Design review of the part built by this model. Coordinates are the model's own, in mm. A direction names the side the tool comes from. Coordinates: 2 decimals unless noted, no trailing zeros. Loops run counter-clockwise (first coordinate to the right, second up) from the corner with the lowest first, then second, coordinate; pieces in that order, holes last. Notation, with made-up numbers: (62, 10) -> (70, 10) arc R20 cw to (70, 49) -> close; hole circle Ø6 at (-11.75, 65.25). An arc over 180 degrees is marked (long way). Use CSV: the item, a comma, the result in double quotes.
```python
from build123d import *

# Parameters (mm, degrees)
BOSS_EXTRUDE1_DEPTH = 15
FILLET1_R           = 5
SKETCH2_W           = 8
SKETCH2_H           = 15
CUT_EXTRUDE1_DEPTH  = 100
SKETCH3_W           = 15
SKETCH3_H           = 70
CUT_EXTRUDE3_DEPTH  = 100
CUT_EXTRUDE4_DEPTH  = 3.75
SKETCH9_R           = 2.5
CUT_EXTRUDE5_DEPTH  = 7.5
SKETCH10_W          = 2.5
SKETCH10_H          = 90
CUT_EXTRUDE6_DEPTH  = 218.431134071
FILLET2_R           = 2
BOSS_EXTRUDE2_DEPTH = 19
SKETCH12_W          = 13.011456799
SKETCH12_H          = 10.932703346
CUT_EXTRUDE7_DEPTH  = 7


with BuildPart() as part:
    # Sketch1 → Boss-Extrude1 (new body)
    with BuildSketch(Plane.XY):
        with BuildLine():
            Line((-15, -103.255813953), (-15, 136.744186047))
            ThreePointArc((-15, 136.744186047), (0, 151.744186047), (15, 136.744186047))
            Line((15, 136.744186047), (140, 136.744186047))
            Line((140, 136.744186047), (140, 111.744186047))
            Line((140, 111.744186047), (15, 111.744186047))
            Line((15, 111.744186047), (15, -103.255813953))
            ThreePointArc((15, -103.255813953), (0, -118.255813953), (-15, -103.255813953))
        make_face()
    extrude(amount=BOSS_EXTRUDE1_DEPTH)

    # Fillet1
    fillet1_edges = [part.edges().sort_by_distance(p)[0] for p in [
        (0, -118.255813953, 0),
        (77.5, 111.744186047, 15),
        (77.5, 136.744186047, 15),
        (0, 151.744186047, 15),
        (-15, 16.744186047, 15),
        (0, -118.255813953, 15),
        (-15, 16.744186047, 0),
        (0, 151.744186047, 0),
        (77.5, 136.744186047, 0),
        (15, 4.244186047, 15),
        (77.5, 111.744186047, 0),
        (15, 4.244186047, 0),
    ]]
    fillet(fillet1_edges, radius=FILLET1_R)

    # Sketch2 → Cut-Extrude1 (cut)
    with BuildSketch(Plane(origin=(140, 0, 0), x_dir=(0, 0, -1), z_dir=(1, 0, 0))):
        with Locations((-7.5, 124.244186047)):
            Rectangle(SKETCH2_W, SKETCH2_H)
    extrude(amount=-CUT_EXTRUDE1_DEPTH, mode=Mode.SUBTRACT)

    # Sketch3 → Cut-Extrude3 (cut)
    with BuildSketch(Plane.XY.offset(15)):
        with Locations((0, -83.255813953)):
            Rectangle(SKETCH3_W, SKETCH3_H)
    extrude(amount=-CUT_EXTRUDE3_DEPTH, mode=Mode.SUBTRACT)

    # Sketch6 → Revolve1 (revolve)
    with BuildSketch(Plane.XY.offset(7.5)):
        with BuildLine():
            Line((-7.5, -101.255813953), (-5.5, -101.255813953))
            ThreePointArc((-5.5, -101.255813953), (-6.085786438, -99.841600391), (-7.5, -99.255813953))
            Line((-7.5, -99.255813953), (-7.5, -101.255813953))
        make_face()
        with BuildLine():
            Line((7.5, -101.255813953), (5.5, -101.255813953))
            ThreePointArc((5.5, -101.255813953), (6.085786438, -99.841600391), (7.5, -99.255813953))
            Line((7.5, -99.255813953), (7.5, -101.255813953))
        make_face()
    revolve(axis=Axis((22.79505848, -101.255813953, 7.5), (-1, 0, 0)))

    # Sketch8 → Cut-Extrude4 (cut, symmetric)
    with BuildSketch(Plane(origin=(0, 0, 0), x_dir=(0, 0, -1), z_dir=(1, 0, 0))):
        Polygon((-7.5, 91.744186047), (0, 86.49262951), (0, 76.49262951), (-7.5, 81.744186047), align=None)
        Polygon((0, 56.49262951), (0, 66.49262951), (-7.5, 71.744186047), (-7.5, 61.744186047), align=None)
        Polygon((0, 36.49262951), (0, 46.49262951), (-7.5, 51.744186047), (-7.5, 41.744186047), align=None)
    extrude(amount=CUT_EXTRUDE4_DEPTH, both=True, mode=Mode.SUBTRACT)

    # Sketch9 → Cut-Extrude5 (cut)
    with BuildSketch(Plane(origin=(0, 0, 0), x_dir=(-1, 0, 0), z_dir=(0, 0, -1))):
        with Locations((-130, 124.244186047)):
            Circle(SKETCH9_R)
        with Locations((-110, 124.244186047)):
            Circle(SKETCH9_R)
        with Locations((-90, 124.244186047)):
            Circle(SKETCH9_R)
        with Locations((-70, 124.244186047)):
            Circle(SKETCH9_R)
        with Locations((-50, 124.244186047)):
            Circle(SKETCH9_R)
    extrude(amount=-CUT_EXTRUDE5_DEPTH, mode=Mode.SUBTRACT)

    # Sketch10 → Cut-Extrude6 (cut, through all)
    with BuildSketch(Plane.ZY.offset(15)):
        with Locations((1.25, -38.255813953)):
            Rectangle(SKETCH10_W, SKETCH10_H)
    extrude(amount=-CUT_EXTRUDE6_DEPTH, mode=Mode.SUBTRACT)

    # Fillet2
    fillet2_edges = [part.edges().sort_by_distance(p)[0] for p in [
        (-12.5, 6.744186047, 0.669872981),
        (12.5, 6.744186047, 0.669872981),
        (8.75, -83.255813953, 0),
        (-8.75, -83.255813953, 0),
        (12.5, -83.255813953, 0.669872981),
        (-12.5, -83.255813953, 0.669872981),
        (0, 6.744186047, 0),
    ]]
    fillet(fillet2_edges, radius=FILLET2_R)

    # Sketch11 → Boss-Extrude2 (add)
    with BuildSketch(Plane.ZY.offset(15)):
        with BuildLine():
            Line((0, 109.244186047), (0, 101.244186047))
            ThreePointArc((0, 101.244186047), (-0.878679656, 103.36550639), (-3, 104.244186047))
            Line((-3, 104.244186047), (-7, 104.244186047))
            Line((-7, 104.244186047), (-7, 109.244186047))
            Line((-7, 109.244186047), (0, 109.244186047))
        make_face()
    extrude(amount=-BOSS_EXTRUDE2_DEPTH)

    # Sketch12 → Cut-Extrude7 (cut)
    with BuildSketch(Plane(origin=(0, 0, -7), x_dir=(-1, 0, 0), z_dir=(0, 0, -1))):
        with Locations((10.2557284, 106.179286635)):
            Rectangle(SKETCH12_W, SKETCH12_H)
    extrude(amount=-CUT_EXTRUDE7_DEPTH, mode=Mode.SUBTRACT)


solid = part.part
```
Item 1: Clearance check with flat-ended pins moving along their axes: pin 1 (4 mm diameter, centred on y = -66, z = 4, fed in from +X); pin 2 (2.5 mm diameter, centred on x = 91.5, z = 6.5, fed in from -Y); pin 3 (3.5 mm diameter, centred on y = 103.5, z = -4, fed in from +X). State where each tip first meets the part, or that it passes through.
Checked values:
pin 1,"x = 15"
pin 2,"y = 111.74"
pin 3,"x = 4"
Item 2: Draft analysis for pull direction Z (two halves, no side actions). For faces 5 (the face through (70.325, 126.723, 1.726)), 6 (the face through (3.75, 44, 4)), 7 (the face through (74.09, 113.17, 1.504)), state which applies: pulls with the +Z half, pulls with the -Z half, needs draft (parallel to the pull), parting line crosses it, or undercut.
Checked values:
face 5,"needs draft"
face 6,"undercut"
face 7,"pulls with the -Z half"
Item 3: Add section A-A (y = -93). Give the boundary of the cut face in (x, z), then the cut area to 3 significant figures.
Checked values:
outline,"(-15, 5) arc R5 ccw to (-10, 0) -> (-7.5, 0) -> (-7.5, 15) -> (-10, 15) arc R5 ccw to (-15, 10) -> close; (7.5, 0) -> (10, 0) arc R5 ccw to (15, 5) -> (15, 10) arc R5 ccw to (10, 15) -> (7.5, 15) -> close"
area,"204 mm^2"
Item 4: Add section B-B (x = 100). Give the boundary of the cut face in (y, z).
Checked values:
outline,"(111.74, 5) arc R5 ccw to (116.74, 0) -> (131.74, 0) arc R5 ccw to (136.74, 5) -> (136.74, 10) arc R5 ccw to (131.74, 15) -> (116.74, 15) arc R5 ccw to (111.74, 10) -> close; hole (116.74, 3.5) -> (131.74, 3.5) -> (131.74, 11.5) -> (116.74, 11.5) -> close"
Item 5: To check wall thickness, follow line 1 along Z through (x, y) = (49.5, 121.5); line 2 along Y through (x, z) = (108, 10); line 3 along Z through (x, y) = (3.5, 44.5). State the ranges of each line that lie inside material, in increasing order.
Checked values:
line 1,"0 to 3.5, 11.5 to 15"
line 2,"111.74 to 116.74, 131.74 to 136.74"
line 3,"7.5 to 15"
Item 6: Add section C-C (x = 22.5). Give the boundary of the cut face in (y, z).
Checked values:
outline,"(111.74, 5) arc R5 ccw to (116.74, 0) -> (131.74, 0) arc R5 ccw to (136.74, 5) -> (136.74, 10) arc R5 ccw to (131.74, 15) -> (116.74, 15) arc R5 ccw to (111.74, 10) -> close"
Item 7: Machinability: for faces 1 (the face through (3.75, 64, 4)), 2 (the face through (140, 124, 12)), 3 (the face through (-0.053, 59.155, 3.802)), 4 (the face through (91, 124, 11.5)), which of the approach directions +Z, -Z, +X, -X, +Y, -Y give a long, thin tool a straight path to every point of the face, cutting with its end or side? Answer none if there is none.
Checked values:
face 1,"none"
face 2,"+Z, -Z, +X, +Y, -Y"
face 3,"-Z"
face 4,"+X"
Item 8: Add section D-D (y = -18). Give the boundary of the cut face in (x, z).
Checked values:
outline,"(-15, 5) arc R5 ccw to (-14.33, 2.5) -> (14.33, 2.5) arc R5 ccw to (15, 5) -> (15, 10) arc R5 ccw to (10, 15) -> (-10, 15) arc R5 ccw to (-15, 10) -> close"
